Read the model definition and answer for the solid it produces. Units are mm, in the model's axes. Face numbers are marked on the shaded views. A direction names the side the tool comes from. Give positions to 0.01 mm unless a question says otherwise; leave off trailing zeros. Order: outer loops, then holes, each group sorted by start corner. A loop starts at its lowest first (then second) coordinate and runs counter-clockwise, first axis right, second up. Notation, with made-up numbers: (84, 44) - (98, 44) arc R21 cw to (98, 61) - close; hole circle Ø3 at (50.25, 85). An arc over 180 degrees is marked (long way). Use a Markdown table: item, result. Add a question column.
1. A cutting plane is placed at A-A on z = -5. Determine the outline of the cut face in (x, y).
2. Consider L1, parallel to Z at x = 9, y = -12.5; L2, parallel to Y at x = 9.5, z = 1; L3, parallel to Y at x = -9, z = 6.75. Determine where each line is inside the solid, lowest interval first.
3. Which of the six approach directions +Z, -Z, +X, -X, +Y, -Y give full straight-line access (tool end or side, diameter ignored) to the marked faces 1 and 2?
4. Flat-ended cylindrical pins translate along their axes: P1, Ø6, axis at y = -7.5, z = -0.5, coming from the +X side; P2, Ø3, axis at y = 0, z = 1, coming from the +X side; P3, Ø5, axis at y = 14, z = 0.5, coming from the +X side. Find the tip coordinate at first contact, or state that the pin passes through.
5. A cutting plane is placed at B-B on z = 3.75. Determine the outline of the cut face in (x, y).
```python
from build123d import *

# Parameters (mm, degrees)
SCHIZZO1_R                   = 11
ESTRUSIONE_ESTRUSIONE1_DEPTH = 7
ESTRUSIONE_ESTRUSIONE2_DEPTH = 8
RACCORDO1_R                  = 1


with BuildPart() as part:
    # Schizzo1 → Estrusione-Estrusione1 (new body)
    with BuildSketch(Plane.XY):
        Circle(SCHIZZO1_R)
    extrude(amount=ESTRUSIONE_ESTRUSIONE1_DEPTH)

    # Schizzo2 → Estrusione-Estrusione2 (add)
    with BuildSketch(Plane(origin=(0, 0, 0), x_dir=(-1, 0, 0), z_dir=(0, 0, -1))):
        Polygon((-19.551988484, -1.747306402), (-8.26278251, -17.806171922), (11.289205974, -16.058865521), (19.551988484, 1.747306402), (8.26278251, 17.806171922), (-11.289205974, 16.058865521), align=None)
    extrude(amount=ESTRUSIONE_ESTRUSIONE2_DEPTH)

    # Raccordo1
    raccordo1_edges = [part.edges().sort_by_distance(p)[0] for p in [
        (15.420597229, 7.155779559, -8),
        (13.907385497, -9.776739162, -8),
        (-1.513211732, -16.932518721, -8),
        (-15.420597229, -7.155779559, -8),
        (-13.907385497, 9.776739162, -8),
        (1.513211732, 16.932518721, -8),
    ]]
    fillet(raccordo1_edges, radius=RACCORDO1_R)


solid = part.part
```
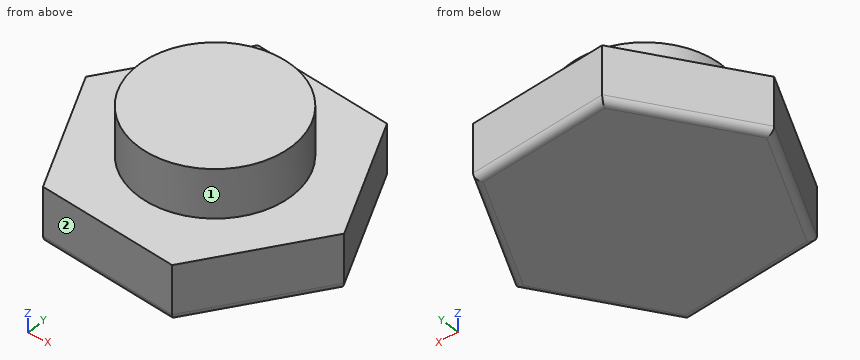
Output values:
| question | item | result |
|---|---|---|
| 1 | outline | (-19.55, 1.75) - (-11.29, -16.06) - (8.26, -17.81) - (19.55, -1.75) - (11.29, 16.06) - (-8.26, 17.81) - close |
| 2 | L1 | -8 to 0 |
| 2 | L2 | -5.55 to 5.55 |
| 2 | L3 | -6.32 to 6.32 |
| 3 | face 1 | +Z |
| 3 | face 2 | +Z, -Z, -X, -Y |
| 4 | P1 | x = 17.62 |
| 4 | P2 | x = 19.26 |
| 4 | P3 | x = 13.38 |
| 5 | outline | circle Ø22 at (0, 0) |
